Design review of the part built by this model. Coordinates are the model's own, in mm. Coordinates: 2 decimals unless noted, no trailing zeros. Loops run counter-clockwise (first coordinate to the right, second up) from the corner with the lowest first, then second, coordinate; pieces in that order, holes last. Notation, with made-up numbers: M 75.25,50.5 L 102.25,50.5 A22 cw 102.25,77.5 Z; hole C 78,-11 d3. An arc over 180 degrees is marked long. Put each result on its own line as item: value. Start each with the question number.
(1) Take a section at A-A, the plane z = 0.8. Give the boundary of the cut face in (x, y) (1 decimal), then the cut area to 3 significant figures.
(2) For probe 1 along X at (y, z) = (-300.5, 2.15); probe 2 along Y at (x, z) = (-31, 1.4); probe 3 along X at (y, z) = (-306.5, 3.5), list the stretches that pass through material, from the lowest coordinate up. Write a range as [from, to].
(3) Take a section at C-C, the plane x = -117. Give the boundary of the cut face in (y, z), then the cut area to 3 significant figures.
(4) Clearance check with flat-ended pins moving along their axes: pin 1 (2.5 mm diameter, centred on y = -305.5, z = 2.5, fed in from -X); pin 2 (2.5 mm diameter, centred on x = 9, z = 2.5, fed in from +Y); pin 3 (1.5 mm diameter, centred on y = -308.5, z = 3, fed in from +X). State where each tip first meets the part, or that it passes through.
(5) Take a section at B-B, the plane y = -333.5. Give the boundary of the cut face in (x, z).
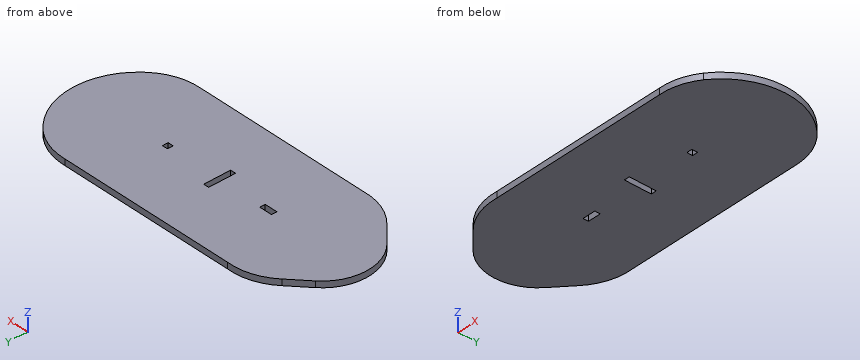
```python
from build123d import *

# Parameters (mm, degrees)
F0_W     = 10
F0_H     = 4.2
F0_W_2   = 4.2
F0_H_2   = 4.413
F0_H_3   = 20.833439
F1_DEPTH = 4.7


with BuildPart() as f1:
    # F0 (on Top) → F1 (new body)
    with BuildSketch(Plane.XY):
        with BuildLine():
            Line((64.647796, -247.966312), (-74.155779, -247.966312))
            ThreePointArc((-74.155779, -247.966312), (-92.018545, -250.466108), (-107.45737, -259.791883))
            Line((-107.45737, -259.791883), (-121.830828, -272.74143))
            ThreePointArc((-121.830828, -272.74143), (-134.169875, -300.46631), (-121.830828, -328.191191))
            Line((-121.830828, -328.191191), (-107.45737, -341.140737))
            ThreePointArc((-107.45737, -341.140737), (-92.018545, -350.466513), (-74.155779, -352.966309))
            Line((-74.155779, -352.966309), (64.647796, -352.966309))
            ThreePointArc((64.647796, -352.966309), (79.384336, -350.969442), (92.668302, -344.284436))
            ThreePointArc((92.668302, -344.284436), (114.427186, -300.46631), (92.668302, -256.648185))
            ThreePointArc((92.668302, -256.648185), (79.384336, -249.963178), (64.647796, -247.966312))
        make_face()
        with Locations((-50.99257, -300.572956)):
            Rectangle(F0_W, F0_H, mode=Mode.SUBTRACT)
        with Locations((34.711947, -300.466456)):
            Rectangle(F0_W_2, F0_H_2, mode=Mode.SUBTRACT)
        with Locations((-9.590311, -300.46631)):
            Rectangle(F0_W_2, F0_H_3, mode=Mode.SUBTRACT)
    extrude(amount=F1_DEPTH)


solid = f1.part
```
Computed values:
1. outline: M -121.8,-328.2 L -107.5,-341.1 A44.9 ccw -74.2,-353 L 64.6,-353 A45.1 ccw 92.7,-344.3 A55 ccw 92.7,-256.6 A45.1 ccw 64.6,-248 L -74.2,-248 A44.9 ccw -107.5,-259.8 L -121.8,-272.7 A37.3 ccw Z; hole M -56,-302.7 L -46,-302.7 L -46,-298.5 L -56,-298.5 Z; hole M -11.7,-310.9 L -7.5,-310.9 L -7.5,-290 L -11.7,-290 Z; hole M 32.6,-302.7 L 36.8,-302.7 L 36.8,-298.3 L 32.6,-298.3 Z
1. area: 23,300 mm^2
2. probe 1: x = [-134.17, -55.99], [-45.99, -11.69], [-7.49, 32.61], [36.81, 114.43]
2. probe 2: y = [-352.97, -247.97]
2. probe 3: x = [-133.68, -11.69], [-7.49, 114.1]
3. outline: M -332.54,0 L -268.39,0 L -268.39,4.7 L -332.54,4.7 Z
3. area: 302 mm^2
4. pin 1: stops at x = -133.98
4. pin 2: stops at y = -247.97
4. pin 3: stops at x = 113.94
5. outline: M -115.94,0 L 103.4,0 L 103.4,4.7 L -115.94,4.7 Z
